```python
from build123d import *

# Parameters (mm, degrees)
SKETCH1_R           = 2.45
BOSS_EXTRUDE1_DEPTH = 5
SKETCH2_R           = 1
BOSS_EXTRUDE2_DEPTH = 2
BOSS_EXTRUDE3_DEPTH = 1


with BuildPart() as part:
    # Sketch1 → Boss-Extrude1 (new body)
    with BuildSketch(Plane(origin=(0, 0, 0), x_dir=(1, 0, 0), z_dir=(0, 1, 0))):
        with BuildLine():
            Line((0, 5), (20, 5))
            Line((20, 5), (20, -5))
            Line((20, -5), (0, -5))
            ThreePointArc((0, -5), (-5, 0), (0, 5))
        make_face()
        Circle(SKETCH1_R, mode=Mode.SUBTRACT)
    extrude(amount=BOSS_EXTRUDE1_DEPTH)

    # Sketch2 → Boss-Extrude2 (add)
    with BuildSketch(Plane(origin=(20, 0, 0), x_dir=(0, 0, -1), z_dir=(1, 0, 0))):
        with BuildLine():
            Line((-5.5, 10), (5.5, 10))
            ThreePointArc((5.5, 10), (8.681980515, 8.681980515), (10, 5.5))
            Line((10, 5.5), (10, 4.5))
            ThreePointArc((10, 4.5), (8.681980515, 1.318019485), (5.5, 0))
            Line((5.5, 0), (-5.5, 0))
            ThreePointArc((-5.5, 0), (-8.681980515, 1.318019485), (-10, 4.5))
            Line((-10, 4.5), (-10, 5.5))
            ThreePointArc((-10, 5.5), (-8.681980515, 8.681980515), (-5.5, 10))
        make_face()
        with Locations((-7.5, 5)):
            Circle(SKETCH2_R, mode=Mode.SUBTRACT)
        with Locations((7.5, 5)):
            Circle(SKETCH2_R, mode=Mode.SUBTRACT)
    extrude(amount=BOSS_EXTRUDE2_DEPTH)

    # Sketch3 → Boss-Extrude3 (add, symmetric)
    with BuildSketch(Plane.XY):
        Polygon((10, 5), (20, 10), (20, 5), align=None)
    extrude(amount=BOSS_EXTRUDE3_DEPTH, both=True)


solid = part.part
```
Could you check a few things on this model? Use its own coordinates, in mm. A direction names the side the tool comes from. Round coordinates to 2 decimals unless told otherwise and drop trailing zeros. Loops run counter-clockwise (first coordinate to the right, second up) from the corner with the lowest first, then second, coordinate; pieces in that order, holes last. Notation, with made-up numbers: (-30.75, -10) - (26.25, -10) arc R16 ccw to (26.25, -2) - close; hole circle Ø9 at (58, 85.25). An arc over 180 degrees is marked (long way). Answer in a Markdown table with one row per item. Add a question column.
(1) If we mould it in two halves opening along X, with no side actions, what happens to faces 6 (the face through (20.986, 8.717, -8.647)), 7 (the face through (14.93, 7.465, 0.014)), 8 (the face through (-0.5, 2.5, 2.4))? For each: pulls with the +X half, pulls with the -X half, needs draft (parallel to the pull), parting line crosses it, or undercut.
(2) For faces 1 (the face through (17, 6, 1)), 2 (the face through (17, 6, -1)), 3 (the face through (10, 2, 5)), 4 (the face through (8, 5, 0)), 5 (the face through (10, 2, -5)), which set-ups out of +Z, -Z, +X, -X, +Y, -Y let a thin tool reach every point of the face, with its end or its side?
(3) If we section it at D-D (x = 4): Please give me the cut outline in (y, z).
(4) I need wall thicknesses on line 1 along Z through (x, y) = (0, 1.5); line 2 along X through (y, z) = (1.35, 0); line 3 along Z through (x, y) = (13, 5.25). Which ranges of each line are inside material? Lowest first, please.
(5) If we section it at C-C (y = 7): Please give me the cut outline in (x, z), plus the area to 3 significant figures.
(6) If we section it at A-A (z = 0): Please give me the cut outline in (x, y).
(7) If we section it at B-B (x = 1): Please give me the cut outline in (y, z).
(8) I'm going to push flat-ended pins straight in: pin 1 (1.5 mm diameter, centred on x = 15, y = 2.5, fed in from +Z); pin 2 (5.5 mm diameter, centred on x = 11.5, y = 3, fed in from -Z); pin 3 (1.5 mm diameter, centred on x = 19, z = 4, fed in from +Y). Where does each tip first touch, or does it pass through?
Model answer:
| question | item | result |
|---|---|---|
| 1 | face 6 | needs draft |
| 1 | face 7 | pulls with the -X half |
| 1 | face 8 | undercut |
| 2 | face 1 | +Z, -X, +Y |
| 2 | face 2 | -Z, -X, +Y |
| 2 | face 3 | +Z, -X, +Y, -Y |
| 2 | face 4 | -X, +Y |
| 2 | face 5 | -Z, -X, +Y, -Y |
| 3 | outline | (0, -5) - (5, -5) - (5, 5) - (0, 5) - close |
| 4 | line 1 | z = -5 to -2.45, 2.45 to 5 |
| 4 | line 2 | x = -5 to -2.45, 2.45 to 22 |
| 4 | line 3 | z = -1 to 1 |
| 5 | outline | (14, -1) - (20, -1) - (20, -9.74) - (22, -9.74) - (22, 9.74) - (20, 9.74) - (20, 1) - (14, 1) - close |
| 5 | area | 51.0 mm² |
| 6 | outline | (-5, 0) - (-2.45, 0) - (-2.45, 5) - (-5, 5) - close; (2.45, 0) - (22, 0) - (22, 10) - (20, 10) - (10, 5) - (2.45, 5) - close |
| 7 | outline | (0, -5) - (5, -5) - (5, -2.24) - (0, -2.24) - close; (0, 2.24) - (5, 2.24) - (5, 5) - (0, 5) - close |
| 8 | pin 1 | stops at z = 5 |
| 8 | pin 2 | stops at z = -5 |
| 8 | pin 3 | stops at y = 5 |
